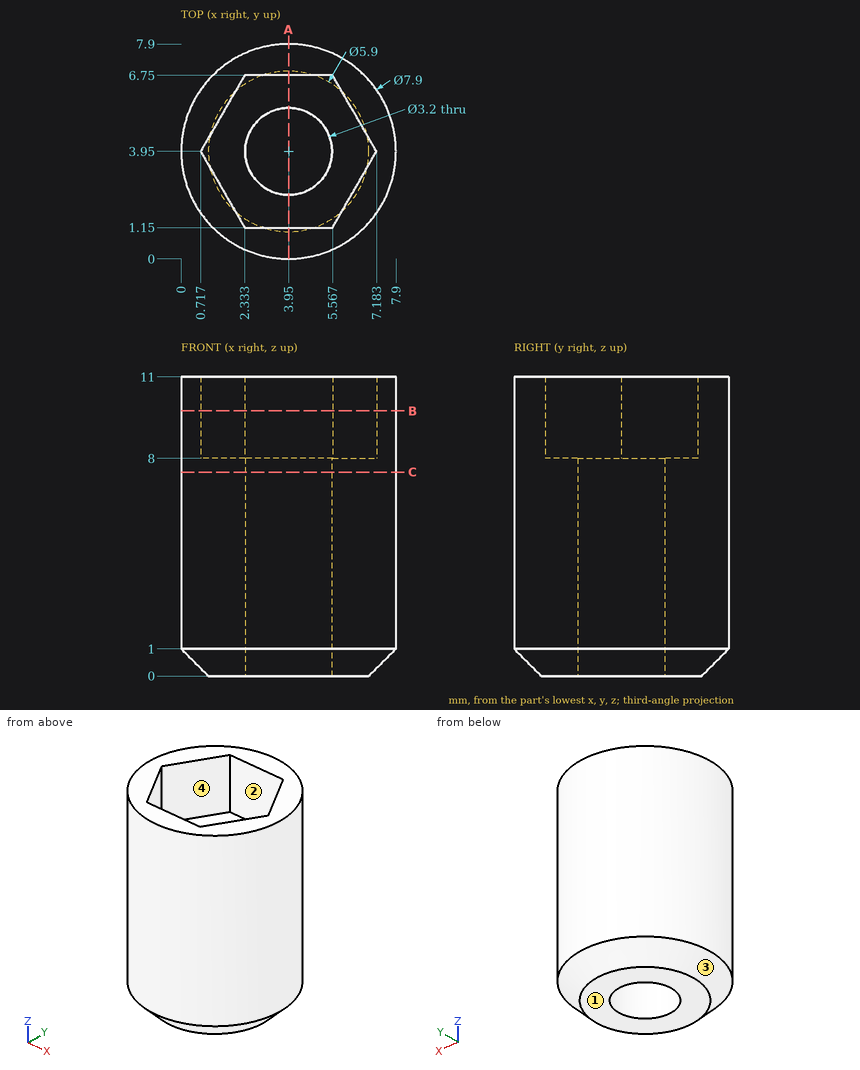
Design review of the part shown in the three views and the two pictorial views. Dimensions are in mm from the part's minimum x, y and z. Round coordinates to 2 decimals unless told otherwise and drop trailing zeros. Loops run counter-clockwise (first coordinate to the right, second up) from the corner with the lowest first, then second, coordinate; pieces in that order, holes last. Notation, with made-up numbers: (-2.5, 51) - (10.5, 51) arc R12 cw to (10.5, 59) - close; hole circle Ø3 at (-17.5, 48). An arc over 180 degrees is marked (long way). Write each question's results on one line, items separated by ' | '. Start each with the question number.
Q1. Wall thickness on line 1 along Y through (x, z) = (3.95, 3.5); line 2 along Z through (x, y) = (1.75, 4); line 3 along Y through (x, z) = (2.75, 8.5): over which ranges is each line inside the solid? List them lowest first. Write a range as [from, to].
Q2. Take a section at C-C on z = 7.5. Give the boundary of the cut face in (x, y).
Q3. Insertion check: P1, Ø1.9, axis at x = 3.95, y = 3.95, coming from the +Z side; P2, Ø1.7, axis at x = 4.5, y = 5, coming from the +Z side; P3, Ø3, axis at x = 2, z = 4, coming from the -Y side; P4, Ø1.5, axis at x = 1, z = 3.5, coming from the -Y side. Each pin has a flat end and moves straight along its axis. Give the tip position at first contact, or say it passes through.
Q4. Take a section at A-A on x = 3.95. Give the boundary of the cut face in (y, z).
Q5. Draft analysis for pull direction Y (two halves, no side actions). For the marked faces 1, 2, 3 and 4, state which applies: pulls with the +Y half, pulls with the -Y half, needs draft (parallel to the pull), parting line crosses it, or undercut.
Q6. Take a section at B-B on z = 9.75. Give the boundary of the cut face in (x, y).
Data:
1) line 1: y = [0, 2.35], [5.55, 7.9] | line 2: z = [0, 8] | line 3: y = [0.19, 1.15], [6.75, 7.71]
2) outline: circle Ø7.9 at (3.95, 3.95); hole circle Ø3.2 at (3.95, 3.95)
3) P1: passes through | P2: stops at z = 8 | P3: stops at y = 0.03 | P4: stops at y = 0.67
4) outline: (0, 1) - (1, 0) - (2.35, 0) - (2.35, 8) - (1.15, 8) - (1.15, 11) - (0, 11) - close; (5.55, 0) - (6.9, 0) - (7.9, 1) - (7.9, 11) - (6.75, 11) - (6.75, 8) - (5.55, 8) - close
5) face 1: needs draft | face 2: undercut | face 3: parting line crosses it | face 4: undercut
6) outline: circle Ø7.9 at (3.95, 3.95); hole (0.72, 3.95) - (2.33, 1.15) - (5.57, 1.15) - (7.18, 3.95) - (5.57, 6.75) - (2.33, 6.75) - close
